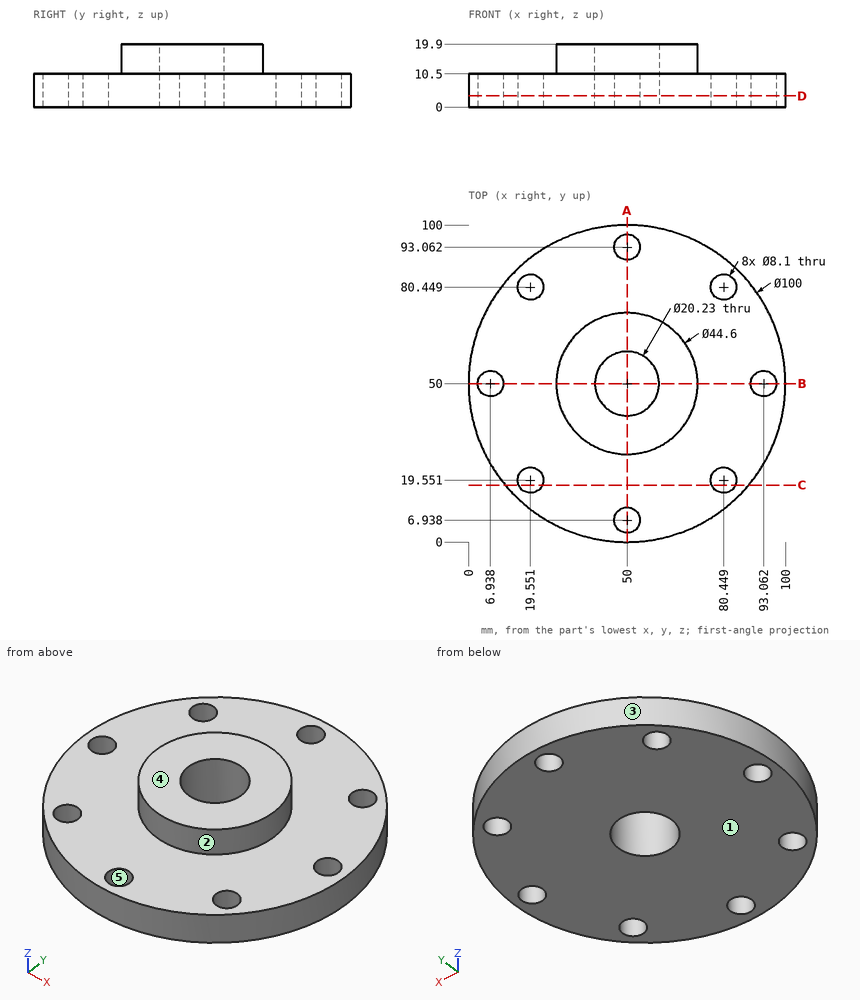
Could you check a few things on this drawing? It's one solid part, dimensions in mm from its lowest x, y, z. A direction names the side the tool comes from. Round coordinates to 2 decimals unless told otherwise and drop trailing zeros. Loops run counter-clockwise (first coordinate to the right, second up) from the corner with the lowest first, then second, coordinate; pieces in that order, holes last. Notation, with made-up numbers: (59, 36.25) -> (103, 36.25) arc R11 ccw to (103, 45.25) -> close; hole circle Ø5 at (27.5, -40). An arc over 180 degrees is marked (long way). Write each question's results on one line, items separated by ' | '.
(1) If we section it at A-A, the plane x = 50: List the corners of the cut face in (y, z) for me (1 decimal).
Worked answers:
outline: (0, 0) -> (2.9, 0) -> (2.9, 10.5) -> (0, 10.5) -> close; (11, 0) -> (39.9, 0) -> (39.9, 19.9) -> (27.7, 19.9) -> (27.7, 10.5) -> (11, 10.5) -> close; (60.1, 0) -> (89, 0) -> (89, 10.5) -> (72.3, 10.5) -> (72.3, 19.9) -> (60.1, 19.9) -> close; (97.1, 0) -> (100, 0) -> (100, 10.5) -> (97.1, 10.5) -> close
(2) If we section it at D-D, the plane z = 3.5: Give the number of separate pieces and of enclosed holes in the cut face, then the cut area to 3 significant figures.
Worked answers:
separate pieces: 1 | enclosed holes: 9 | area: 7,120 mm2
(3) If I drill on L1, parallel to Y at x = 50, z = 6 (1 decimal); L2, parallel to Z at x = 14.5, y = 75.5; L3, parallel to Y at x = 41.5, z = 14.75 (1 decimal), over which ranges is the centre line in solid material (lowest first)?
Worked answers:
L1: 0 to 2.9, 11 to 39.9, 60.1 to 89, 97.1 to 100 | L2: 0 to 10.5 | L3: 29.4 to 44.5, 55.5 to 70.6
(4) We'd pull the mould along X, two halves only. Please class the marked faces 3, 4 and 5: released by +X, released by -X, zero draft, split by the parting line, or undercut.
Worked answers:
face 3: split by the parting line | face 4: zero draft | face 5: undercut
(5) For P1, Ø5, axis at x = 65, z = 14.5, coming from the -Y side; P2, Ø10, axis at y = 38.5, z = 13, coming from the +X side; P3, Ø9.5, axis at x = 80.45, y = 19.55, coming from the +Z side, each with a flat end and sliding along its axis, tell me the tip position at first contact or that it passes through.
Worked answers:
P1: y = 31.53 | P2: x = 99.48 | P3: z = 10.5
(6) If we section it at C-C, the plane y = 18: List the corners of the cut face in (x, z) for me.
Worked answers:
outline: (11.58, 0) -> (15.81, 0) -> (15.81, 10.5) -> (11.58, 10.5) -> close; (23.29, 0) -> (76.71, 0) -> (76.71, 10.5) -> (23.29, 10.5) -> close; (84.19, 0) -> (88.42, 0) -> (88.42, 10.5) -> (84.19, 10.5) -> close
(7) For the marked faces 1 and 2, which set-ups out of +Z, -Z, +X, -X, +Y, -Y let a thin tool reach every point of the face, with its end or its side?
Worked answers:
face 1: -Z, +X, -X, +Y, -Y | face 2: +Z
